Source: CAD feature listing. Evaluate the final solid. Frame: model axes, mm. A direction names the side the tool comes from. Give positions to 0.01 mm unless a question says otherwise; leave off trailing zeros. Order: outer loops, then holes, each group sorted by start corner. A loop starts at its lowest first (then second) coordinate and runs counter-clockwise, first axis right, second up. Notation, with made-up numbers: (36, -25) -> (68, -25) arc R17 cw to (68, -20) -> close; hole circle Ø1 at (-39, 3). An arc over 180 degrees is marked (long way). Answer in a Markdown table with one row per item.
```python
from build123d import *

# Parameters (mm, degrees)
SCHIZZO1_R                   = 8
ESTRUSIONE_ESTRUSIONE1_DEPTH = 40
SCHIZZO2_R                   = 40
ESTRUSIONE_ESTRUSIONE2_DEPTH = 5
SCHIZZO3_R                   = 6
ESTRUSIONE_ESTRUSIONE3_DEPTH = 230
SCHIZZO4_W                   = 4
SCHIZZO4_H                   = 20
TAGLIO_ESTRUSIONE1_DEPTH     = 281.757902827
RACCORDO1_R                  = 4


with BuildPart() as part:
    # Schizzo1 → Estrusione-Estrusione1 (new body)
    with BuildSketch(Plane(origin=(0, 0, 0), x_dir=(1, 0, 0), z_dir=(0, 1, 0))):
        with Locations(Location((0, 0, 0), (0, 0, 270))):
            Circle(SCHIZZO1_R)
    extrude(amount=ESTRUSIONE_ESTRUSIONE1_DEPTH)

    # Schizzo2 → Estrusione-Estrusione2 (add)
    with BuildSketch(Plane(origin=(0, 40, 0), x_dir=(1, 0, 0), z_dir=(0, 1, 0))):
        with Locations(Location((0, 0, 0), (0, 0, 270))):
            Circle(SCHIZZO2_R)
    extrude(amount=ESTRUSIONE_ESTRUSIONE2_DEPTH)

    # Schizzo3 → Estrusione-Estrusione3 (add)
    with BuildSketch(Plane(origin=(0, 45, 0), x_dir=(1, 0, 0), z_dir=(0, 1, 0))):
        with Locations(Location((0, 0, 0), (0, 0, 270))):
            Circle(SCHIZZO3_R)
    extrude(amount=ESTRUSIONE_ESTRUSIONE3_DEPTH)

    # Schizzo4 → Taglio-Estrusione1 (cut, symmetric)
    with BuildSketch(Plane.XY):
        with Locations((6, 10)):
            Rectangle(SCHIZZO4_W, SCHIZZO4_H)
    taglio_estrusione1 = extrude(amount=TAGLIO_ESTRUSIONE1_DEPTH, both=True, mode=Mode.SUBTRACT)

    # Specchia1: Taglio-Estrusione1 across plane
    add(taglio_estrusione1.mirror(Plane(origin=(0, 0, 0), x_dir=(0, 0, 1), z_dir=(1, 0, 0))), mode=Mode.SUBTRACT)


with BuildPart() as body_2:
    # Schizzo5 → Rivoluzione1 (revolve)
    with BuildSketch(Plane(origin=(0, 0, 0), x_dir=(0, 0, -1), z_dir=(1, 0, 0))):
        with BuildLine():
            Line((-6, 8), (6, 8))
            ThreePointArc((6, 8), (0, 14), (-6, 8))
        make_face()
    revolve(axis=Axis((0, 8, 6), (0, 0, -1)))


with BuildPart() as part_1:
    add(part.part)

    # Abbina1: cut body 2
    add(body_2.part, mode=Mode.SUBTRACT)

    # Raccordo1
    # the kernel refuses this fillet: 4 mm, written as the material it adds along each edge
    with BuildSketch(Plane(origin=(4, 20, 16.92820323), x_dir=(0, -1, 0), z_dir=(0, 0, -1))) as raccordo1_piece_1_section:
        with BuildLine():
            CenterArc((RACCORDO1_R, -RACCORDO1_R), RACCORDO1_R, 90, 90)
            Line((0, -RACCORDO1_R), (0, 0))
            Line((0, 0), (RACCORDO1_R, 0))
        make_face()
    raccordo1_piece_1 = extrude(amount=33.856406461, mode=Mode.PRIVATE)
    raccordo1_piece_1 = raccordo1_piece_1 & Plane(origin=(0, 19.029808041, 0), x_dir=(0, 0, 1), z_dir=(0, -1, 0)) * Cylinder(8, 84, mode=Mode.PRIVATE)
    add(raccordo1_piece_1)
    with BuildSketch(Plane(origin=(-4, 20, 16.92820323), x_dir=(0, -1, 0), z_dir=(0, 0, -1))) as raccordo1_piece_2_section:
        with BuildLine():
            CenterArc((RACCORDO1_R, RACCORDO1_R), RACCORDO1_R, 180, 90)
            Line((0, RACCORDO1_R), (0, 0))
            Line((0, 0), (RACCORDO1_R, 0))
        make_face()
    raccordo1_piece_2 = extrude(amount=33.856406461, mode=Mode.PRIVATE)
    raccordo1_piece_2 = raccordo1_piece_2 & Plane(origin=(0, 19.029808041, 0), x_dir=(0, 0, 1), z_dir=(0, -1, 0)) * Cylinder(8, 84, mode=Mode.PRIVATE)
    add(raccordo1_piece_2)
    # the kernel refuses this fillet: 4 mm, written as the material it takes off along each edge
    with BuildSketch(Plane(origin=(-4, 0, 16.92820323), x_dir=(1, 0, 0), z_dir=(0, 0, -1))) as raccordo1_2_piece_1:
        with BuildLine():
            CenterArc((RACCORDO1_R, -RACCORDO1_R), RACCORDO1_R, 90, 90)
            Line((0, -RACCORDO1_R), (0, 0))
            Line((0, 0), (RACCORDO1_R, 0))
        make_face()
    extrude(amount=33.856406461, mode=Mode.SUBTRACT)
    with BuildSketch(Plane(origin=(4, 0, 16.92820323), x_dir=(-1, 0, 0), z_dir=(0, 0, -1))) as raccordo1_2_piece_2:
        with BuildLine():
            CenterArc((RACCORDO1_R, RACCORDO1_R), RACCORDO1_R, 180, 90)
            Line((0, RACCORDO1_R), (0, 0))
            Line((0, 0), (RACCORDO1_R, 0))
        make_face()
    extrude(amount=33.856406461, mode=Mode.SUBTRACT)


solid = part_1.part
```
(1) Section query A-A (y = 137). Return the cut outline in (x, z).
A:
| item | result |
|---|---|
| outline | circle Ø12 at (0, 0) |
(2) Section query B-B (z = 17). Return the cut outline in (x, y), plus the area to 3 significant figures.
A:
| item | result |
|---|---|
| outline | (-36.21, 40) -> (36.21, 40) -> (36.21, 45) -> (-36.21, 45) -> close |
| area | 362 mm^2 |
(3) Access query for faces 1 (the flat face through (4, 13, 0)), 2 (the cylindrical face through (1.802, 158.39, 5.723)), 3 (the flat face through (-4, 13, 0)). Directions: +Z, -Z, +X, -X, +Y, -Y. A direction counts if a zero-diameter tool reaches every point of the face in a straight line with its end or side. Return the directions, or none.
A:
| item | result |
|---|---|
| face 1 | +Z, -Z, +X, -Y |
| face 2 | +Y |
| face 3 | +Z, -Z, -X, -Y |
(4) Section query C-C (x = -26.5). Return the cut outline in (y, z).
A:
| item | result |
|---|---|
| outline | (40, -29.96) -> (45, -29.96) -> (45, 29.96) -> (40, 29.96) -> close |
(5) Ray query, probe 1 along Z at (x, y) = (-4.5, 166.5); probe 2 along Y at (x, z) = (0.5, 21.5); probe 3 along Z at (x, y) = (1.5, 53). Return the intervals inside material, ascending.
A:
| item | result |
|---|---|
| probe 1 | z = -3.97 to 3.97 |
| probe 2 | y = 40 to 45 |
| probe 3 | z = -5.81 to 5.81 |
(6) First-contact query: pin 1 Ø3 at (x, z) = (0.5, 30.5) entering from -Y; pin 2 Ø13 at (y, z) = (7, 1) entering from +X; pin 3 Ø3 at (x, z) = (-13, 15) entering from +Y. Flat tips, straight axial feed; report the tip coordinate or a pass-through.
A:
| item | result |
|---|---|
| pin 1 | stops at y = 40 |
| pin 2 | stops at x = 4 |
| pin 3 | stops at y = 45 |
